Here's how the part is built. I have some questions about the finished solid (model axes, mm). A direction names the side the tool comes from. Round coordinates to 2 decimals unless told otherwise and drop trailing zeros. Loops run counter-clockwise (first coordinate to the right, second up) from the corner with the lowest first, then second, coordinate; pieces in that order, holes last. Notation, with made-up numbers: (13, -39) -> (35, -39) arc R25 ccw to (35, -20) -> close; hole circle Ø11 at (28, -17.75). An arc over 180 degrees is marked (long way). Use CSV: the item, a comma, the result in double quotes. Start each with the question number.
from build123d import *

# Parameters (mm, degrees)
SKETCH1_R           = 77.1
BOSS_EXTRUDE1_DEPTH = 8
SKETCH2_R           = 2.25
CUT_EXTRUDE1_DEPTH  = 110.328953164
SKETCH3_R           = 3
CUT_EXTRUDE2_DEPTH  = 5
SKETCH4_R           = 12
CUT_EXTRUDE3_DEPTH  = 5
SKETCH5_R           = 9
CUT_EXTRUDE4_DEPTH  = 5


with BuildPart() as part:
    # Sketch1 → Boss-Extrude1 (new body)
    with BuildSketch(Plane(origin=(0, 0, 0), x_dir=(1, 0, 0), z_dir=(0, 1, 0))):
        with Locations(Location((0, 0, 0), (0, 0, 270))):
            Circle(SKETCH1_R)
    extrude(amount=BOSS_EXTRUDE1_DEPTH)

    # Sketch2 → Cut-Extrude1 (cut, through all)
    with BuildSketch(Plane(origin=(0, 8, 0), x_dir=(1, 0, 0), z_dir=(0, 1, 0))):
        with Locations(Location((0, 71.8, 0), (0, 0, 270))):
            Circle(SKETCH2_R)
        with Locations(Location((50.770266889, 50.770266889, 0), (0, 0, 270))):
            Circle(SKETCH2_R)
        with Locations(Location((71.8, 0, 0), (0, 0, 270))):
            Circle(SKETCH2_R)
        with Locations(Location((50.770266889, -50.770266889, 0), (0, 0, 270))):
            Circle(SKETCH2_R)
        with Locations(Location((0, -71.8, 0), (0, 0, 270))):
            Circle(SKETCH2_R)
        with Locations(Location((-50.770266889, -50.770266889, 0), (0, 0, 270))):
            Circle(SKETCH2_R)
        with Locations(Location((-71.8, 0, 0), (0, 0, 270))):
            Circle(SKETCH2_R)
        with Locations(Location((-50.770266889, 50.770266889, 0), (0, 0, 270))):
            Circle(SKETCH2_R)
    extrude(amount=-CUT_EXTRUDE1_DEPTH, mode=Mode.SUBTRACT)

    # Sketch3 → Cut-Extrude2 (cut)
    with BuildSketch(Plane.XZ):
        with Locations(Location((60, 0, 0), (0, 0, 270))):
            Circle(SKETCH3_R)
        with Locations(Location((57.955549577, -15.529142706, 0), (0, 0, 270))):
            Circle(SKETCH3_R)
        with Locations(Location((51.961524227, -30, 0), (0, 0, 270))):
            Circle(SKETCH3_R)
        with Locations(Location((42.426406871, -42.426406871, 0), (0, 0, 270))):
            Circle(SKETCH3_R)
        with Locations(Location((30, -51.961524227, 0), (0, 0, 270))):
            Circle(SKETCH3_R)
        with Locations(Location((15.529142706, -57.955549577, 0), (0, 0, 270))):
            Circle(SKETCH3_R)
        with Locations(Location((0, -60, 0), (0, 0, 270))):
            Circle(SKETCH3_R)
        with Locations(Location((-15.529142706, -57.955549577, 0), (0, 0, 270))):
            Circle(SKETCH3_R)
        with Locations(Location((-30, -51.961524227, 0), (0, 0, 270))):
            Circle(SKETCH3_R)
        with Locations(Location((-42.426406871, -42.426406871, 0), (0, 0, 270))):
            Circle(SKETCH3_R)
        with Locations(Location((-51.961524227, -30, 0), (0, 0, 270))):
            Circle(SKETCH3_R)
        with Locations(Location((-57.955549577, -15.529142706, 0), (0, 0, 270))):
            Circle(SKETCH3_R)
        with Locations(Location((-60, 0, 0), (0, 0, 270))):
            Circle(SKETCH3_R)
        with Locations(Location((-57.955549577, 15.529142706, 0), (0, 0, 270))):
            Circle(SKETCH3_R)
        with Locations(Location((-51.961524227, 30, 0), (0, 0, 270))):
            Circle(SKETCH3_R)
        with Locations(Location((-42.426406871, 42.426406871, 0), (0, 0, 270))):
            Circle(SKETCH3_R)
        with Locations(Location((-30, 51.961524227, 0), (0, 0, 270))):
            Circle(SKETCH3_R)
        with Locations(Location((-15.529142706, 57.955549577, 0), (0, 0, 270))):
            Circle(SKETCH3_R)
        with Locations(Location((0, 60, 0), (0, 0, 270))):
            Circle(SKETCH3_R)
        with Locations(Location((15.529142706, 57.955549577, 0), (0, 0, 270))):
            Circle(SKETCH3_R)
        with Locations(Location((30, 51.961524227, 0), (0, 0, 270))):
            Circle(SKETCH3_R)
        with Locations(Location((42.426406871, 42.426406871, 0), (0, 0, 270))):
            Circle(SKETCH3_R)
        with Locations(Location((51.961524227, 30, 0), (0, 0, 270))):
            Circle(SKETCH3_R)
        with Locations(Location((57.955549577, 15.529142706, 0), (0, 0, 270))):
            Circle(SKETCH3_R)
    extrude(amount=-CUT_EXTRUDE2_DEPTH, mode=Mode.SUBTRACT)

    # Sketch4 → Cut-Extrude3 (cut)
    with BuildSketch(Plane(origin=(0, 8, 0), x_dir=(1, 0, 0), z_dir=(0, 1, 0))):
        with Locations(Location((0, 0, 0), (0, 0, 270))):
            Circle(SKETCH4_R)
    extrude(amount=-CUT_EXTRUDE3_DEPTH, mode=Mode.SUBTRACT)

    # Sketch5 → Cut-Extrude4 (cut)
    with BuildSketch(Plane(origin=(0, 3, 0), x_dir=(1, 0, 0), z_dir=(0, 1, 0))):
        with Locations(Location((0, 0, 0), (0, 0, 270))):
            Circle(SKETCH5_R)
    extrude(amount=-CUT_EXTRUDE4_DEPTH, mode=Mode.SUBTRACT)


solid = part.part
Q1. Will these pins go through, and if not, where does the flat tip stop? pin 1 Ø1.5 at (x, y) = (59.5, 5) entering from +Z; pin 2 Ø5.5 at (x, z) = (57.96, -15.53) entering from -Y; pin 3 Ø1.5 at (y, z) = (3.5, 50.5) entering from -X; pin 4 Ø2 at (x, z) = (22, 35) entering from -Y.
Q2. I want a section at D-D, the plane x = 71.8. List the corners of the cut face in (y, z) for me.
Q3. I want a section at C-C, the plane z = -71.8. List the corners of the cut face in (x, y) for me.
Q4. For faces 1 (the cylindrical face through (30.13, 2.46, 54.96)), 2 (the cylindrical face through (-69.57, 4.06, -0.29)), which set-ups out of +Z, -Z, +X, -X, +Y, -Y let a thin tool reach every point of the face, with its end or its side?
Q5. I want a section at A-A, the plane x = 0. List the corners of the cut face in (y, z) for me.
Q6. I want a section at B-B, the plane z = 0. List the corners of the cut face in (x, y) for me, then the cut area to 3 significant figures.
Q7. I need wall thicknesses on line 1 along Z through (x, y) = (-58, 3); line 2 along Z through (x, y) = (43, 1.5); line 3 along Z through (x, y) = (-56, 2.25). Which ranges of each line are inside material? Lowest first, please.
Values found:
1,pin 1,"z = 49.93"
1,pin 2,"y = 5"
1,pin 3,"x = -58.9"
1,pin 4,"y = 0"
2,outline,"(0, -28.09) -> (8, -28.09) -> (8, -2.25) -> (0, -2.25) -> close; (0, 2.25) -> (8, 2.25) -> (8, 28.09) -> (0, 28.09) -> close"
3,outline,"(-28.09, 0) -> (-2.25, 0) -> (-2.25, 8) -> (-28.09, 8) -> close; (2.25, 0) -> (28.09, 0) -> (28.09, 8) -> (2.25, 8) -> close"
4,face 1,"-Y"
4,face 2,"+Y, -Y"
5,outline,"(0, -77.1) -> (8, -77.1) -> (8, -74.05) -> (0, -74.05) -> close; (0, -69.55) -> (8, -69.55) -> (8, -12) -> (3, -12) -> (3, -9) -> (0, -9) -> (0, -57) -> (5, -57) -> (5, -63) -> (0, -63) -> close; (0, 9) -> (3, 9) -> (3, 12) -> (8, 12) -> (8, 69.55) -> (0, 69.55) -> (0, 63) -> (5, 63) -> (5, 57) -> (0, 57) -> close; (0, 74.05) -> (8, 74.05) -> (8, 77.1) -> (0, 77.1) -> close"
6,outline,"(-77.1, 0) -> (-74.05, 0) -> (-74.05, 8) -> (-77.1, 8) -> close; (-69.55, 0) -> (-63, 0) -> (-63, 5) -> (-57, 5) -> (-57, 0) -> (-9, 0) -> (-9, 3) -> (-12, 3) -> (-12, 8) -> (-69.55, 8) -> close; (9, 0) -> (57, 0) -> (57, 5) -> (63, 5) -> (63, 0) -> (69.55, 0) -> (69.55, 8) -> (12, 8) -> (12, 3) -> (9, 3) -> close; (74.05, 0) -> (77.1, 0) -> (77.1, 8) -> (74.05, 8) -> close"
6,area,"928 mm2"
7,line 1,"-50.8 to -18.53, -12.53 to -2.24, 2.24 to 12.53, 18.53 to 50.8"
7,line 2,"-64 to -45.37, -39.48 to 39.48, 45.37 to 64"
7,line 3,"-52.99 to -17.8, -13.25 to 13.25, 17.8 to 52.99"
